```python
from build123d import *

# Parameters (mm, degrees)
RESSALTO_EXTRUS_O1_DEPTH = 120
CORTE_EXTRUS_O1_DEPTH    = 40


with BuildPart() as part:
    # Esboço2 → Ressalto-extrusão1 (new body)
    with BuildSketch(Plane.XY):
        Polygon((15, 8.660254038), (0, 17.320508076), (-15, 8.660254038), (-15, -8.660254038), (0, -17.320508076), (15, -8.660254038), align=None)
    extrude(amount=RESSALTO_EXTRUS_O1_DEPTH)

    # Esboço1 → Corte-extrusão1 (cut)
    with BuildSketch(Plane.XY):
        Polygon((9, 5.196152423), (0, 10.392304845), (-9, 5.196152423), (-9, -5.196152423), (0, -10.392304845), (9, -5.196152423), align=None)
    extrude(amount=CORTE_EXTRUS_O1_DEPTH, mode=Mode.SUBTRACT)


solid = part.part
```
Check sheet for the modelled part. Datum: model origin and axes. Units: mm. A direction names the side the tool comes from. Coordinates: 2 decimals unless noted, no trailing zeros. Write each loop counter-clockwise with the first axis right and the second up, starting at its lowest first coordinate (ties: lowest second). Pieces come first, ordered by that corner, then holes. Notation, with made-up numbers: M 85.25,35 L 144.25,35 A16 cw 144.25,50 Z; hole C -11,27.25 d6. An arc over 180 degrees is marked long. Write item = value, one per line. Start each with the question number.
1. Mould release check, pull along Y, two halves, no side actions. Record for faces 1 (the flat face through (7.605, 12.93, 59.16)), 2 (the flat face through (-4.44, 7.83, 19.72)), 3 (the flat face through (7.4, -13.05, 59.16)): pulls with the +Y half, pulls with the -Y half, needs draft (parallel to the pull), parting line crosses it, or undercut.
2. Sectioned sample at B-B (y = 0.5). Record the cut outline in (x, z).
3. Sectioned sample at C-C (x = 6). Record the cut outline in (y, z), then the cut area to 3 significant figures.
4. Go/stop test with flat-tipped pins: pin 1 (6 mm diameter, centred on x = 6.5, z = 20, fed in from +Y); pin 2 (4 mm diameter, centred on x = 1, z = 81.5, fed in from -Y); pin 3 (5.5 mm diameter, centred on x = -3.5, y = -4.5, fed in from -Z). Record where each tip stops, or that it passes through.
5. Thickness scan on probe 1 along Z at (x, y) = (-5.5, 7); probe 2 along Y at (x, z) = (-4.25, 39); probe 3 along X at (y, z) = (-6, 11.5). Record the ranges inside material, lowest first.
6. Sectioned sample at D-D (z = 49.5). Record the cut outline in (x, y), then the cut area to 3 significant figures.
7. Tool access check on faces 4 (the flat face through (4.44, -7.83, 19.72)), 5 (the flat face through (-7, -7, 0)). Record the directions out of +Z, -Z, +X, -X, +Y, -Y that give a thin tool (end or side, any length) a straight path to the whole face; none if there is none.
8. Sectioned sample at A-A (z = 17). Record the cut outline in (x, y).
The answers:
q1.face_1 = pulls with the +Y half
q1.face_2 = undercut
q1.face_3 = pulls with the -Y half
q2.outline = M -15,0 L -9,0 L -9,40 L 9,40 L 9,0 L 15,0 L 15,120 L -15,120 Z
q3.outline = M -13.86,0 L -6.93,0 L -6.93,40 L 6.93,40 L 6.93,0 L 13.86,0 L 13.86,120 L -13.86,120 Z
q3.area = 2,770 mm²
q4.pin_1 = 15.3
q4.pin_2 = -17.32
q4.pin_3 = 40
q5.probe_1 = 40 to 120
q5.probe_2 = -14.87 to -7.94, 7.94 to 14.87
q5.probe_3 = -15 to -7.61, 7.61 to 15
q6.outline = M -15,-8.66 L 0,-17.32 L 15,-8.66 L 15,8.66 L 0,17.32 L -15,8.66 Z
q6.area = 779 mm²
q7.face_4 = -Z
q7.face_5 = -Z, +X, -X, +Y, -Y
q8.outline = M -15,-8.66 L 0,-17.32 L 15,-8.66 L 15,8.66 L 0,17.32 L -15,8.66 Z; hole M -9,-5.2 L 0,-10.39 L 9,-5.2 L 9,5.2 L 0,10.39 L -9,5.2 Z
